Autodesk Inventor part; units mm, degrees
ref_plane "YZ Plane" through (0, 0, 0) normal (1, 0, 0) x (0, 1, 0)
ref_plane "XZ Plane" through (0, 0, 0) normal (0, 1, 0) x (-1, 0, 0)
ref_plane "XY Plane" through (0, 0, 0) normal (0, 0, 1) x (1, 0, 0)
sketch "Sketch1" plane through (0, 0, 0) normal (0, 1, 0) x (-1, 0, 0)
  line L0 (-165, 65) -> (165, 65)
  line L1 (165, 65) -> (165, -65)
  line L2 (165, -65) -> (-165, -65)
  line L3 (-165, -65) -> (-165, 65)
  line L4 (-165, 65) -> (165, -65) construction
  line L5 (165, 65) -> (-165, -65) construction
  point P0 (0, 0)
  dimension "d0" = 330
  dimension "d1" = 130
extrude "Extrusion1" add sketch "Sketch1" along normal blind 25
sketch "Sketch2" plane through (0, 25, 0) normal (0, 1, 0) x (1, 0, 0)
  line L0 (160.5, -60.5) -> (-160.5, -60.5)
  line L1 (-160.5, -60.5) -> (-160.5, 60.5)
  line L2 (-160.5, 60.5) -> (160.5, 60.5)
  line L3 (160.5, 60.5) -> (160.5, -60.5)
  line L4 (160.5, -60.5) -> (-160.5, 60.5) construction
  line L5 (-160.5, -60.5) -> (160.5, 60.5) construction
  point P0 (0, 0)
  dimension "d4" = 321
  dimension "d5" = 121
extrude "Extrusion2" cut sketch "Sketch2" against normal blind 20
fillet "Fillet1" radius 2 4 edges at (-160.5, 15, -60.5) (160.5, 15, -60.5) (-160.5, 15, 60.5) (160.5, 15, 60.5)
properties part number "Shelf V2"
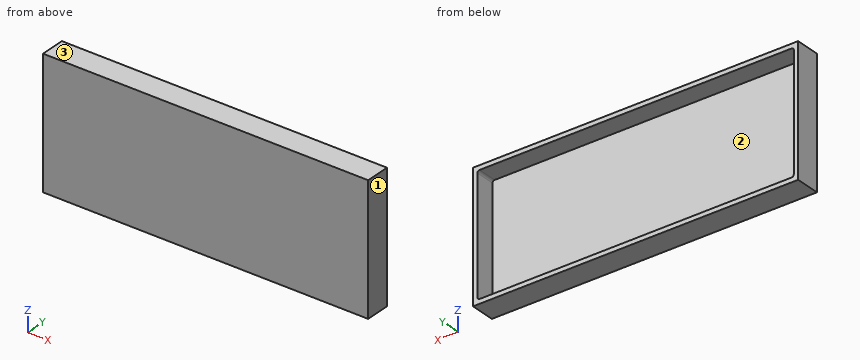
Could you check a few things on this model? Use its own coordinates, in mm. Face numbers are marked on the shaded views. Coordinates: 2 decimals unless noted, no trailing zeros. Order: outer loops, then holes, each group sorted by start corner. A loop starts at its lowest first (then second) coordinate and runs counter-clockwise, first axis right, second up.
Q1. Will this pin go through, and if not, where does the flat tip stop? pin 1 (12 mm diameter, centred on x = 63.5, z = -46.5, fed in from +Y).
Q2. Suppose I cut it at A-A on y = 15.75. Please give me the cut outline in (x, z).
Q3. Suppose I cut it at B-B on x = -36. Please give me the cut outline in (y, z), and give its area (3 significant figures).
Q4. Thinking about a two-plate mould opening in X: for the marked faces 1, 2 and 3, which applies, released by +X, released by -X, zero draft, split by the parting line, or undercut?
Q5. Please list where these lines run through material, in increasing order: L1, parallel to Z at x = -113.5, y = 5.75; L2, parallel to X at y = 18, z = -38; L3, parallel to Y at x = 134, z = 55.5.
Q6. Suppose I cut it at C-C on z = 51. Please give me the cut outline in (x, y).
Answer:
1. pin 1: stops at y = 5
2. outline: (-165, -65) - (165, -65) - (165, 65) - (-165, 65) - close; hole (-160.5, -58.5) arc R2 ccw to (-158.5, -60.5) - (158.5, -60.5) arc R2 ccw to (160.5, -58.5) - (160.5, 58.5) arc R2 ccw to (158.5, 60.5) - (-158.5, 60.5) arc R2 ccw to (-160.5, 58.5) - close
3. outline: (0, -65) - (25, -65) - (25, -60.5) - (5, -60.5) - (5, 60.5) - (25, 60.5) - (25, 65) - (0, 65) - close
3. area: 830 mm2
4. face 1: released by +X
4. face 2: undercut
4. face 3: zero draft
5. L1: z = -65 to -60.5, 60.5 to 65
5. L2: x = -165 to -160.5, 160.5 to 165
5. L3: y = 0 to 5
6. outline: (-165, 0) - (165, 0) - (165, 25) - (160.5, 25) - (160.5, 5) - (-160.5, 5) - (-160.5, 25) - (-165, 25) - close
